Model file for the job. Use its own axes, mm. Face numbers are marked on the shaded views. A direction names the side the tool comes from. Round coordinates to 2 decimals unless told otherwise and drop trailing zeros. Write each loop counter-clockwise with the first axis right and the second up, starting at its lowest first coordinate (ties: lowest second). Pieces come first, ordered by that corner, then holes. Notation, with made-up numbers: (59.5, 64.25) - (65.5, 64.25) arc R25 ccw to (65.5, 96.25) - close; hole circle Ø11 at (-27.75, 23). An arc over 180 degrees is marked (long way). One line per item, written item: value.
from build123d import *

# Parameters (mm, degrees)
FILLET1_R = 2


with BuildPart() as part:
    # Sketch1 → Revolve1 (revolve)
    with BuildSketch(Plane.XY, mode=Mode.PRIVATE) as revolve1_sk:
        with BuildLine():
            Line((-16, 7), (16, 7))
            Line((16, 7), (16, 13))
            Line((16, 13), (14, 13))
            Line((14, 13), (14, 23))
            Line((14, 23), (7, 23))
            ThreePointArc((7, 23), (0, 16), (-7, 23))
            Line((-7, 23), (-14, 23))
            Line((-14, 23), (-14, 13))
            Line((-14, 13), (-16, 13))
            Line((-16, 13), (-16, 7))
        make_face()
    revolve(revolve1_sk.sketch.rotate(Axis((0, 0, 0), (-1, 0, 0)), 90), axis=Axis((0, 0, 0), (-1, 0, 0)))

    # Fillet1
    fillet1_edges = [part.edges().sort_by_distance(p)[0] for p in [
        (-14, 0, 13),
        (14, 0, 13),
    ]]
    fillet(fillet1_edges, radius=FILLET1_R - 0.0001)  # a hair under: the kernel refuses the full size


solid = part.part
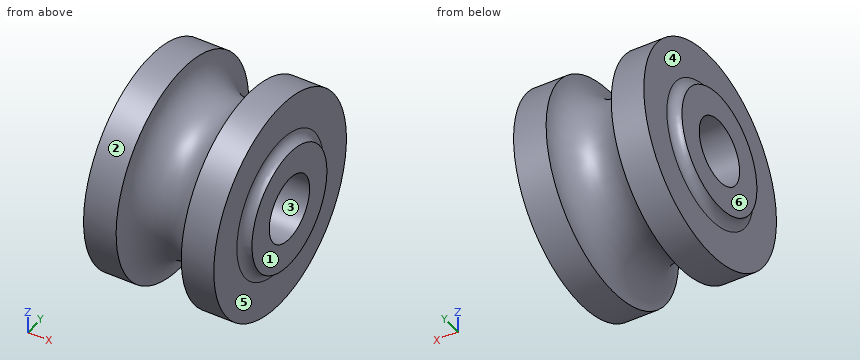
1. Band-saw the part on C-C on x = -13. Write the cut outline in (y, z).
Report:
outline: circle Ø46 at (0, 0); hole circle Ø14 at (0, 0)
2. Band-saw the part on D-D on x = 4.5. Write the cut outline in (y, z), plus the area to 3 significant figures.
Report:
outline: circle Ø35.28 at (0, 0); hole circle Ø14 at (0, 0)
area: 823 mm²
3. Wall check: probe 1 along Y at (x, z) = (8, 0); probe 2 along Z at (x, y) = (-8, 3); probe 3 along X at (y, z) = (18, -14). Give the ranges that are in metal, low to high. Write a range as [from, to].
Report:
probe 1: [-23, -7], [7, 23]
probe 2: [-22.8, -6.32], [6.32, 22.8]
probe 3: [-14, -7], [7, 14]
4. Tool access for the marked faces 4, 5 and 6: list every direction of +Z, -Z, +X, -X, +Y, -Y with a clear straight run to the whole face (end or side of a thin tool).
Report:
face 4: -X
face 5: +X
face 6: +Z, -Z, -X, +Y, -Y
5. Drop flat-ended pins along their axis: pin 1 (1.5 mm diameter, centred on x = 10, z = -13.5, fed in from +Y); pin 2 (10 mm diameter, centred on x = 0, z = -0.5, fed in from -Y); pin 3 (4 mm diameter, centred on x = 6, z = 14, fed in from -Y) (3 decimals); pin 4 (8.5 mm diameter, centred on y = 0, z = 0, fed in from +X) (3 decimals). Give the stop position or say it passes through.
Report:
pin 1: y = 19.14
pin 2: y = -18.1
pin 3: y = -19.455
pin 4: through
6. Mould opens along Z. For the marked faces 1, 2 and 3 say: released by +Z, released by -Z, zero draft, split by the parting line, or undercut.
Report:
face 1: zero draft
face 2: split by the parting line
face 3: undercut
